from build123d import *

# Parameters (mm, degrees)
F0_R          = 8.7929686237
F1_DEPTH      = 25.4
F2_R          = 4.9489279231
F3_DEPTH      = 43.18
F3_DEPTH_BACK = 43.18
F5_DEPTH      = 25.4
F5_DEPTH_BACK = 25.4


with BuildPart() as f1:
    # F0 (on Top) → F1 (new body)
    with BuildSketch(Plane.XY):
        with BuildLine():
            ThreePointArc((-20.5612275749, -70.7723498344), (0, -91.3335774094), (20.5612275749, -70.7723498344))
            Line((20.5612275749, -70.7723498344), (20.5612275749, 70.7723498344))
            ThreePointArc((20.5612275749, 70.7723498344), (0, 91.3335774094), (-20.5612275749, 70.7723498344))
            Line((-20.5612275749, 70.7723498344), (-20.5612275749, -70.7723498344))
        make_face()
        with Locations((0, -70.7723498344)):
            Circle(F0_R, mode=Mode.SUBTRACT)
        with Locations((0, 70.7723498344)):
            Circle(F0_R, mode=Mode.SUBTRACT)
    extrude(amount=F1_DEPTH)

    # F2 (on Front) → F3 (join, two sides)
    with BuildSketch(Plane.XZ) as f3_sk:
        with BuildLine():
            Line((-12.5674372539, 25.4), (0, 25.4))
            Line((0, 25.4), (12.5674372539, 25.4))
            Line((12.5674372539, 25.4), (12.5674372539, 60.96))
            ThreePointArc((12.5674372539, 60.96), (0, 73.5274372539), (-12.5674372539, 60.96))
            Line((-12.5674372539, 60.96), (-12.5674372539, 25.4))
        make_face()
        with Locations((0, 60.96)):
            Circle(F2_R, mode=Mode.SUBTRACT)
    extrude(amount=F3_DEPTH)
    extrude(f3_sk.sketch, amount=-F3_DEPTH_BACK)

    # F4 (on Right) → F5 (cut, two sides)
    with BuildSketch(Plane.YZ) as f5_sk:
        with BuildLine():
            Line((23.6512031406, 93.859386313), (-23.6512031406, 93.859386313))
            Line((-23.6512031406, 93.859386313), (-23.6512031406, 43.059386313))
            ThreePointArc((-23.6512031406, 43.059386313), (0, 30.9874073241), (23.6512031406, 43.059386313))
            Line((23.6512031406, 43.059386313), (23.6512031406, 93.859386313))
        make_face()
    extrude(amount=-F5_DEPTH, mode=Mode.SUBTRACT)
    extrude(f5_sk.sketch, amount=F5_DEPTH_BACK, mode=Mode.SUBTRACT)


solid = f1.part
Could you check a few things on this model? Use its own coordinates, in mm. A direction names the side the tool comes from. Give positions to 0.01 mm unless a question says otherwise; leave off trailing zeros. Order: outer loops, then holes, each group sorted by start corner. A loop starts at its lowest first (then second) coordinate and runs counter-clockwise, first axis right, second up. Notation, with made-up numbers: (-12.5, 82.5) - (12.5, 82.5) arc R22 ccw to (12.5, 118.5) - close; hole circle Ø10 at (64.5, 56.5). An arc over 180 degrees is marked (long way). One line per question, with ' | ' between items. Start each with the question number.
Item 1: I want a section at C-C on x = 0. Write out the boundary of the cut face in (y, z), then the cut area to 3 significant figures.
Item 2: I want a section at B-B on z = 52.5. Write out the boundary of the cut face in (x, y), then the cut area to 3 significant figures.
Item 3: I need wall thicknesses on probe 1 along Y at (x, z) = (0, 19); probe 2 along Z at (x, y) = (0, 37.75); probe 3 along X at (y, z) = (37.75, 60.96). Which ranges of each line are inside material? Lowest first, please. Write a range as [from, to].
Item 4: Thinking about a two-plate mould opening in Y: for faces 1 (the cylindrical face through (-0.45, -91.33, 12.52)), 2 (the cylindrical face through (-1.91, 62.19, 12.52)), 3 (the flat face through (-20.561, 1, 13)), 4 (the flat face through (0, 23.651, 55)), which applies, pulls with the +Y half, pulls with the -Y half, needs draft (parallel to the pull), parting line crosses it, or undercut?
Item 5: For faces 5 (the flat face through (-12.567, -1, 28)), 6 (the flat face through (0, 43.18, 50)), 7 (the flat face through (13, 1, 25.4)), 8 (the flat face through (12.567, -1, 27)), which set-ups out of +Z, -Z, +X, -X, +Y, -Y let a thin tool reach every point of the face, with its end or its side?
Item 6: I want a section at A-A on y = 32. Write out the boundary of the cut face in (x, z), then the cut area to 3 significant figures.
Item 7: I want a section at D-D on z = 11.5. Write out the boundary of the cut face in (x, y), then the cut area to 3 significant figures.
Item 8: I'm going to push flat-ended pins straight in: pin 1 Ø6 at (x, z) = (10.5, 33.5) entering from -Y; pin 2 Ø3 at (x, z) = (12, 7.5) entering from -Y; pin 3 Ø12.5 at (x, z) = (4, 51) entering from +Y; pin 4 Ø4 at (x, y) = (0, -13) entering from -Z. Where does each tip first touch, or does it pass through?
Verdict:
1) outline: (-91.33, 0) - (-79.57, 0) - (-79.57, 25.4) - (-91.33, 25.4) - close; (-61.98, 0) - (61.98, 0) - (61.98, 25.4) - (43.18, 25.4) - (43.18, 56.01) - (23.65, 56.01) - (23.65, 43.06) arc R29.2 cw to (-23.65, 43.06) - (-23.65, 56.01) - (-43.18, 56.01) - (-43.18, 25.4) - (-61.98, 25.4) - close; (-43.18, 65.91) - (-23.65, 65.91) - (-23.65, 73.53) - (-43.18, 73.53) - close; (23.65, 65.91) - (43.18, 65.91) - (43.18, 73.53) - (23.65, 73.53) - close; (79.57, 0) - (91.33, 0) - (91.33, 25.4) - (79.57, 25.4) - close | area: 5,680 mm^2
2) outline: (-12.57, -43.18) - (12.57, -43.18) - (12.57, -23.65) - (-12.57, -23.65) - close; (-12.57, 23.65) - (12.57, 23.65) - (12.57, 43.18) - (-12.57, 43.18) - close | area: 982 mm^2
3) probe 1: [-91.33, -79.57], [-61.98, 61.98], [79.57, 91.33] | probe 2: [0, 56.01], [65.91, 73.53] | probe 3: [-12.57, -4.95], [4.95, 12.57]
4) face 1: pulls with the -Y half | face 2: undercut | face 3: needs draft | face 4: undercut
5) face 5: +Z, -X, +Y, -Y | face 6: +Z, +X, -X, +Y | face 7: +Z | face 8: +Z, +X, +Y, -Y
6) outline: (-20.56, 0) - (20.56, 0) - (20.56, 25.4) - (12.57, 25.4) - (12.57, 60.96) arc R12.57 ccw to (-12.57, 60.96) - (-12.57, 25.4) - (-20.56, 25.4) - close; hole circle Ø9.9 at (0, 60.96) | area: 2,110 mm^2
7) outline: (-20.56, -70.77) arc R20.56 ccw to (20.56, -70.77) - (20.56, 70.77) arc R20.56 ccw to (-20.56, 70.77) - close; hole circle Ø17.59 at (0, -70.77); hole circle Ø17.59 at (0, 70.77) | area: 6,660 mm^2
8) pin 1: y = -43.18 | pin 2: y = -88.45 | pin 3: y = 43.18 | pin 4: z = 0
